Work out the finished part from the listing and answer in its coordinate system (mm). A direction names the side the tool comes from. Coordinates: 2 decimals unless noted, no trailing zeros. Loops run counter-clockwise (first coordinate to the right, second up) from the corner with the lowest first, then second, coordinate; pieces in that order, holes last. Notation, with made-up numbers: (-20, 81.25) -> (10, 81.25) arc R22 ccw to (10, 119.25) -> close; hole circle Ø8 at (-28, -37). An arc over 180 degrees is marked (long way). Use a Markdown table: item, result.
from build123d import *

# Parameters (mm, degrees)
SKETCH_1_R          = 5
EXTRUDE_1_DEPTH     = 6
FILLET_1_R          = 10
SKETCH_4_W          = 37
SKETCH_4_H          = 3
EXTRUDE_2_DEPTH     = 30
SKETCH_5_W          = 6
SKETCH_5_H          = 1.5
EXTRUDE_3_DEPTH     = 30
SKETCH_6_R          = 1.6
CUT_EXTRUDE_1_DEPTH = 10
EXTRUDE_5_DEPTH     = 15
SKETCH_10_R         = 1.75
CUT_EXTRUDE_3_DEPTH = 1000
EXTRUDE_6_DEPTH     = 15


with BuildPart() as part:
    # Эскиз1 → Бобышка-Вытянуть1 (new body)
    with BuildSketch(Plane.XY):
        Polygon((0, 0), (0, 65), (16, 65), (21, 65), (37, 65), (37, 0), align=None)
        with Locations((18.5, 43)):
            Circle(SKETCH_1_R, mode=Mode.SUBTRACT)
    extrude(amount=EXTRUDE_1_DEPTH)

    # Скругление1
    fillet_1_edges = [part.edges().sort_by_distance(p)[0] for p in [
        (0, 65, 3),
        (37, 65, 3),
    ]]
    fillet(fillet_1_edges, radius=FILLET_1_R)

    # Эскиз4 → Бобышка-Вытянуть2 (add)
    with BuildSketch(Plane.XY.offset(6)):
        with Locations((18.5, -1.5)):
            Rectangle(SKETCH_4_W, SKETCH_4_H)
    extrude(amount=-EXTRUDE_2_DEPTH)

    # Эскиз5 → Бобышка-Вытянуть3 (add)
    with BuildSketch(Plane.XY.offset(6)):
        with Locations((18.5, -3.75)):
            Rectangle(SKETCH_5_W, SKETCH_5_H)
    extrude(amount=-EXTRUDE_3_DEPTH)

    # Эскиз6 → Вырез-Вытянуть1 (cut)
    with BuildSketch(Plane.XY.offset(6)):
        with Locations((3, 27.5)):
            Circle(SKETCH_6_R)
        with Locations((3, 58.5)):
            Circle(SKETCH_6_R)
        with Locations((34, 27.5)):
            Circle(SKETCH_6_R)
        with Locations((34, 58.5)):
            Circle(SKETCH_6_R)
    extrude(amount=-CUT_EXTRUDE_1_DEPTH, mode=Mode.SUBTRACT)

    # Эскиз9 → Бобышка-Вытянуть5 (add)
    with BuildSketch(Plane.ZY):
        Polygon((-24, 0), (0, 0), (0, 15.416167011), align=None)
    extrude(amount=-EXTRUDE_5_DEPTH)

    # Эскиз10 → Вырез-Вытянуть3 (cut)
    with BuildSketch(Plane.XZ.offset(4.5)):
        with Locations((18.5, -18)):
            Circle(SKETCH_10_R)
        with Locations((18.425804873, -4)):
            Circle(SKETCH_10_R)
    extrude(amount=-CUT_EXTRUDE_3_DEPTH, mode=Mode.SUBTRACT)

    # Эскиз11 → Бобышка-Вытянуть6 (add)
    with BuildSketch(Plane(origin=(37, 0, 0), x_dir=(0, 0, -1), z_dir=(1, 0, 0))):
        Polygon((0, 0), (24, 0), (0, 15.416167011), align=None)
    extrude(amount=-EXTRUDE_6_DEPTH)


solid = part.part
Q1. Section A-A on y = 43 is taken. Determine the outline of the cut face in (x, z), and give its area (3 significant figures).
Solved:
| item | result |
|---|---|
| outline | (0, 0) -> (13.5, 0) -> (13.5, 6) -> (0, 6) -> close; (23.5, 0) -> (37, 0) -> (37, 6) -> (23.5, 6) -> close |
| area | 162 mm² |
Q2. Given pin 1 Ø10 at (x, y) = (12, 20) entering from -Z; pin 2 Ø6 at (x, y) = (9, 20) entering from -Z; pin 3 Ø17 at (x, z) = (32, -16.5) entering from -Y, each flat-ended and moving along its own axis, determine where each tip first touches the part or whether it passes through.
Solved:
| item | result |
|---|---|
| pin 1 | z = -0.65 |
| pin 2 | z = 0 |
| pin 3 | y = -3 |
Q3. Section B-B on z = -18 is taken. Determine the outline of the cut face in (x, y), and give its area (3 significant figures).
Solved:
| item | result |
|---|---|
| outline | (0, -3) -> (15.5, -3) -> (15.5, -4.5) -> (16.75, -4.5) -> (16.75, 0) -> (15, 0) -> (15, 3.85) -> (0, 3.85) -> close; (20.25, -4.5) -> (21.5, -4.5) -> (21.5, -3) -> (37, -3) -> (37, 3.85) -> (22, 3.85) -> (22, 0) -> (20.25, 0) -> close |
| area | 220 mm² |
Q4. For faces 4 (the flat face through (18, 0, -12)), 5 (the flat face through (21.5, -4, -9)), 6 (the flat face through (8, -3, -9)), 7 (the cylindrical face through (2.85, 61.99, 3.04)), determine the directions among +Z, -Z, +X, -X, +Y, -Y from which every point of the face is accessible in a straight line to the end or side of a thin tool.
Solved:
| item | result |
|---|---|
| face 4 | -Z, +Y |
| face 5 | +Z, -Z, +X, -Y |
| face 6 | +Z, -Z, -X, -Y |
| face 7 | +Z, -Z, -X, +Y |
Q5. Section D-D on z = 0.75 is taken. Determine the outline of the cut face in (x, y).
Solved:
| item | result |
|---|---|
| outline | (0, -3) -> (15.5, -3) -> (15.5, -4.5) -> (21.5, -4.5) -> (21.5, -3) -> (37, -3) -> (37, 55) arc R10 ccw to (27, 65) -> (10, 65) arc R10 ccw to (0, 55) -> close; hole circle Ø3.2 at (3, 27.5); hole circle Ø3.2 at (3, 58.5); hole circle Ø10 at (18.5, 43); hole circle Ø3.2 at (34, 27.5); hole circle Ø3.2 at (34, 58.5) |
Q6. Consider line 1 (Z direction, x = 18.5, y = -1.65); line 2 (Y direction, x = 34, z = 2.5); line 3 (X direction, y = 6.5, z = -2.5). Determine where each line is inside the solid, lowest interval first. Write a range as [from, to].
Solved:
| item | result |
|---|---|
| line 1 | [-24, -19.75], [-16.25, -5.75], [-2.25, 6] |
| line 2 | [-3, 25.9], [29.1, 56.9], [60.1, 62.14] |
| line 3 | [0, 15], [22, 37] |
Q7. Section C-C on x = 34 is taken. Determine the outline of the cut face in (y, z).
Solved:
| item | result |
|---|---|
| outline | (-3, -24) -> (0, -24) -> (15.42, 0) -> (25.9, 0) -> (25.9, 6) -> (-3, 6) -> close; (29.1, 0) -> (56.9, 0) -> (56.9, 6) -> (29.1, 6) -> close; (60.1, 0) -> (62.14, 0) -> (62.14, 6) -> (60.1, 6) -> close |
Q8. Determine the mould class of faces 1 (the flat face through (15.5, -4, -9)), 2 (the flat face through (18, -2, -24)), 3 (the cylindrical face through (20.042, -2.282, -4.67)) for opening direction Z: pulls with the +Z half, pulls with the -Z half, needs draft (parallel to the pull), parting line crosses it, or undercut.
Solved:
| item | result |
|---|---|
| face 1 | needs draft |
| face 2 | pulls with the -Z half |
| face 3 | undercut |
